Design review of the part built by this model. Coordinates are the model's own, in mm. Face numbers are marked on the shaded views. A direction names the side the tool comes from. Coordinates: 2 decimals unless noted, no trailing zeros. Loops run counter-clockwise (first coordinate to the right, second up) from the corner with the lowest first, then second, coordinate; pieces in that order, holes last.
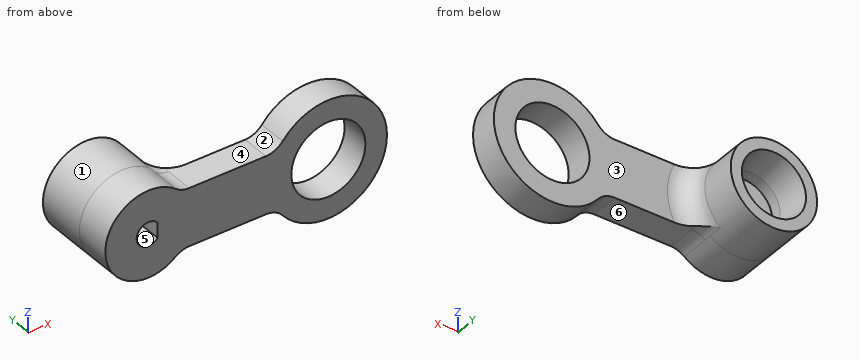
Autodesk Inventor part; units mm, degrees
ref_plane "YZ Plane" through (0, 0, 0) normal (1, 0, 0) x (0, 1, 0)
ref_plane "XZ Plane" through (0, 0, 0) normal (0, 1, 0) x (-1, 0, 0)
ref_plane "XY Plane" through (0, 0, 0) normal (0, 0, 1) x (1, 0, 0)
sketch "Boceto1" plane through (0, 0, 0) normal (0, 1, 0) x (-1, 0, 0)
  circle A0 centre (0, 0) radius 4
  circle A1 centre (0, 0) radius 1.65
  line L0 (0, 4) -> (-25, 4)
  line L1 (-25, 4) -> (-25, -4)
  line L2 (-25, -4) -> (0, -4)
  line L3 (0, -4) -> (0, 4)
  circle A2 centre (-25, 0) radius 4
  circle A3 centre (-25, 0) radius 1.65
  line L4 (-1.27, 1.0534) -> (-1.27, -1.0534)
  point P0 (-25, 4)
  point P1 (0, -4)
  dimension "d1" = 8
  dimension "d0" = 3.3
  dimension "d2" = 25
  dimension "d3" = 3.3
  dimension "d4" = 1.27
extrude "Extrusión1" add sketch "Boceto1" along normal blind 5 contours A0 L3 A1 | L3 A1 A0 | A0 L2 A2 L0 | A2 L1 A3 | L1 A3 A2 | L4 A1
sketch "Boceto5" plane through (0, 5, 0) normal (0, 1, 0) x (1, 0, 0)
  circle A0 centre (0, 0) radius 6
  dimension "d12" = 12
extrude "Extrusión4" add sketch "Boceto5" along normal blind 7
sketch "Boceto8" plane through (0, 12, 0) normal (0, 1, 0) x (1, 0, 0)
  circle A0 centre (0, 0) radius 3.95
  dimension "d21" = 7.9
extrude "Extrusión5" cut sketch "Boceto8" against normal blind 4.26
sketch "Boceto9" plane through (0, 0, 0) normal (0, -1, 0) x (1, 0, 0)
  arc A0 (4.4721, 4) -> (4.4721, -4) centre (0, 0) ccw
  arc A1 (4.4721, -4) -> (4.4721, 4) centre (0, 0) ccw
  line L0 (25, -4) -> (0, -4)
  arc A2 (25, -4) -> (25, 4) centre (25, 0) ccw
  line L1 (0, 4) -> (25, 4)
  arc A3 (0, 4) -> (0, -4) centre (0, 0) ccw
  arc A4 (1.27, 1.0534) -> (1.27, -1.0534) centre (0, 0) ccw
  line L2 (1.27, -1.0534) -> (1.27, 1.0534)
  circle A5 centre (25, 0) radius 1.65
  point P0 (4.4721, 4)
  point P1 (4.4721, -4)
extrude "Extrusión6" add sketch "Boceto9" against normal up to surface (5 mm away) contours L1 A3 L0 A0
sketch "Boceto10" plane through (0, 12, 0) normal (0, 1, 0) x (1, 0, 0)
  circle A0 centre (0, 0) radius 4.45
  dimension "d26" = 8.9
loft "Solevación2" cut profiles "Boceto10" section 2 edges at (-3.95, 7.74, 0)
sketch "Boceto11" plane through (0, 7.74, 0) normal (0, 1, 0) x (1, 0, 0)
  circle A0 centre (0, 0) radius 3.95
extrude "Extrusión7" cut sketch "Boceto11" against normal blind 1.5
sketch "Boceto12" plane through (0, 5, 0) normal (0, 1, 0) x (1, 0, 0)
  arc A0 (4.4721, -4) -> (4.4721, 4) centre (0, 0) ccw
  line L0 (4.4721, -4) -> (25, -4)
  arc A1 (25, -4) -> (25, 4) centre (25, 0) ccw
  line L1 (25, 4) -> (4.4721, 4)
  circle A2 centre (25, 0) radius 1.65
extrude "Extrusión8" cut sketch "Boceto12" against normal blind 1
sketch "Boceto14" plane through (0, 4, 0) normal (0, 1, 0) x (1, 0, 0)
  circle A0 centre (25, 0) radius 1.65
  circle A1 centre (25, 0) radius 5.15
  circle A2 centre (25, 0) radius 8.15
  point P0 (0, 0)
  dimension "d36" = 10.3
  dimension "d37" = 3
extrude "Extrusión9" add sketch "Boceto14" against normal up to surface (4 mm away) contours A2
sketch "Boceto15" plane through (0, 4, 0) normal (0, 1, 0) x (1, 0, 0)
  arc A0 (21.7562, -4) -> (21.7562, 4) centre (25, 0) ccw
  circle A1 centre (25, 0) radius 5.15
  point P0 (0, 0)
  point P1 (21.7562, 4)
  dimension "d35" = 17.0679
extrude "Extrusión10" cut sketch "Boceto15" against normal through all
fillet "Empalme1" radius 3 5 edges at (17.8991, 2, 4) (17.8991, 2, -4) (4.4721, 2, -4) (4.4721, 2, 4) (6, 4, 0)
sketch "Boceto6" plane through (0, 12, 0) normal (0, 1, 0) x (1, 0, 0)
  circle A0 centre (0, 0) radius 4.5
  dimension "d15" = 9
sketch "Boceto7" plane through (0, 5, 0) normal (0, 1, 0) x (1, 0, 0)
  arc A0 (1.27, 1.0534) -> (1.27, -1.0534) centre (0, 0) ccw
  circle A1 centre (0, 0) radius 4
  dimension "d16" = 8
sketch "Boceto2" plane through (0, 5, 0) normal (0, 1, 0) x (1, 0, 0)
  line L0 (40, 3) -> (0, 3)
  arc A0 (0, 3) -> (0, -3) centre (0, 0) ccw
  line L1 (0, -3) -> (40, -3)
  arc A1 (40, -3) -> (40, 3) centre (40, 0) ccw
  arc A2 (1.27, 1.0534) -> (1.27, -1.0534) centre (0, 0) ccw
  line L2 (1.27, 1.0534) -> (1.27, -1.0534)
  circle A3 centre (40, 0) radius 1.65
sketch "Boceto4" plane through (0, 6.2, 0) normal (0, 1, 0) x (1, 0, 0)
  arc A0 (1.27, 1.0534) -> (1.27, -1.0534) centre (0, 0) ccw
  circle A1 centre (0, 0) radius 5
  dimension "d9" = 10
properties part number "LinkA"
Q1. Take a section at B-B, the plane y = 2.75. Write out the cut boundary in (x, z), then the cut area to 3 significant figures.
Q2. The part is to be moulded in two halves that separate along X. For the marked faces 1, 2 and 3, say which applies: pulls with the +X half, pulls with the -X half, needs draft (parallel to the pull), parting line crosses it, or undercut.
Q3. Take a section at C-C, the plane x = 0. Write out the cut boundary in (y, z).
Q4. For line 1 (X direction, y = 1.2, z = 0); line 2 (Z direction, x = 0, y = 7.2); line 3 (Z direction, x = 0, y = 1.5), list the stretches that pass through material, from the lowest coordinate up.
Q5. Clearance check with flat-ended pins moving along their axes: pin 1 Ø1.4 at (x, y) = (9.5, 3) entering from -Z; pin 2 Ø6 at (x, z) = (25, 0) entering from -Y; pin 3 Ø1.5 at (x, z) = (16.5, -4) entering from +Y; pin 4 Ø1.5 at (x, y) = (3, 1.5) entering from +Z. State where each tip first meets the part, or that it passes through.
Q6. Take a section at D-D, the plane z = 7.25. Write out the cut boundary in (x, y).
Q7. Take a section at A-A, the plane x = 25. Write out the cut boundary in (y, z), then the cut area to 3 significant figures.
Q8. Machinability: for the marked faces 4, 5 and 6, which of the approach directions +Z, -Z, +X, -X, +Y, -Y give a long, thin tool a straight path to every point of the face, cutting with its end or side? Answer none if there is none.
Entries:
1. outline: (3.77, -4.67) arc R3 cw to (5.66, -4) - (16.32, -4) arc R3 cw to (18.66, -5.12) arc R8.15 ccw (long way) to (18.66, 5.12) arc R3 cw to (16.32, 4) - (5.66, 4) arc R3 cw to (3.77, 4.67) arc R6 ccw (long way) to start; hole (1.27, -1.05) - (1.27, 1.05) arc R1.65 ccw (long way) to start; hole circle Ø10.3 at (25, 0)
1. area: 325 mm2
2. face 1: parting line crosses it
2. face 2: undercut
2. face 3: needs draft
3. outline: (0, -6) - (12, -6) - (12, -4.45) - (7.74, -3.95) - (6.24, -3.95) - (6.24, 3.95) - (7.74, 3.95) - (12, 4.45) - (12, 6) - (0, 6) - (0, 1.65) - (5, 1.65) - (5, -1.65) - (0, -1.65) - close
4. line 1: x = -6 to -1.65, 1.27 to 19.85, 30.15 to 33.15
4. line 2: z = -6 to -3.95, 3.95 to 6
4. line 3: z = -6 to -1.65, 1.65 to 6
5. pin 1: stops at z = -4
5. pin 2: passes through
5. pin 3: stops at y = 4
5. pin 4: stops at z = 5.56
6. outline: (21.28, 0) - (28.72, 0) - (28.72, 4) - (21.28, 4) - close
7. outline: (0, -8.15) - (4, -8.15) - (4, -5.15) - (0, -5.15) - close; (0, 5.15) - (4, 5.15) - (4, 8.15) - (0, 8.15) - close
7. area: 24.0 mm2
8. face 4: +Z, +Y, -Y
8. face 5: -Y
8. face 6: -Z, +Y, -Y
